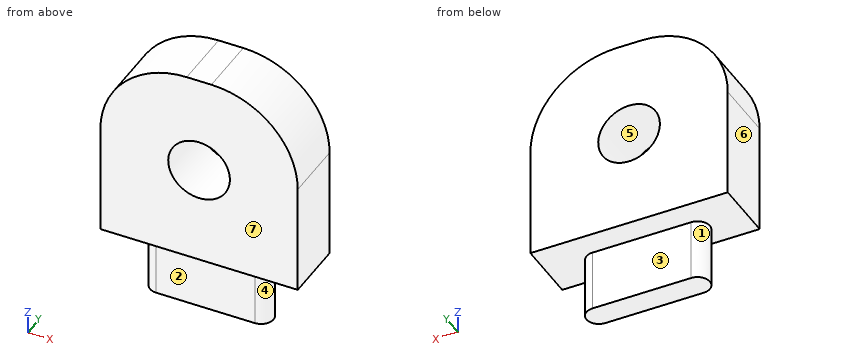
from build123d import *

# Parameters (mm, degrees)
SKETCH1_R           = 2.5
BOSS_EXTRUDE1_DEPTH = 5
BOSS_EXTRUDE2_DEPTH = 5


with BuildPart() as part:
    # Sketch1 → Boss-Extrude1 (new body)
    with BuildSketch(Plane(origin=(0, 0, 0), x_dir=(1, 0, 0), z_dir=(0, 1, 0))):
        with BuildLine():
            Line((-8, 0), (-8, -9))
            ThreePointArc((-8, -9), (-5.949747468, -13.949747468), (-1, -16))
            Line((-1, -16), (1, -16))
            ThreePointArc((1, -16), (5.949747468, -13.949747468), (8, -9))
            Line((8, -9), (8, 0))
            Line((8, 0), (-8, 0))
        make_face()
        with Locations(Location((0, -8, 0), (0, 0, 270))):
            Circle(SKETCH1_R, mode=Mode.SUBTRACT)
    extrude(amount=BOSS_EXTRUDE1_DEPTH)

    # Sketch2 → Boss-Extrude2 (add)
    with BuildSketch(Plane(origin=(0, 0, 0), x_dir=(-1, 0, 0), z_dir=(0, 0, -1))):
        with BuildLine():
            Line((-4, 3), (4, 3))
            ThreePointArc((4, 3), (5, 2), (4, 1))
            Line((4, 1), (-4, 1))
            ThreePointArc((-4, 1), (-5, 2), (-4, 3))
        make_face()
    extrude(amount=BOSS_EXTRUDE2_DEPTH)


solid = part.part
Could you check a few things on this model? Use its own coordinates, in mm. Face numbers are marked on the shaded views. A direction names the side the tool comes from. Coordinates: 2 decimals unless noted, no trailing zeros. Order: outer loops, then holes, each group sorted by start corner. A loop starts at its lowest first (then second) coordinate and runs counter-clockwise, first axis right, second up.
Q1. Suppose I cut it at C-C on x = 1.25. Please give me the cut outline in (y, z).
Q2. Which directions (+Z, -Z, +X, -X, +Y, -Y) give clear straight access to the entire face, cutting with the end or side of a thin tool? Please do the marked faces 1, 2 and 3.
Q3. Suppose I cut it at D-D on z = 5.75. Please give me the cut outline in (x, y).
Q4. Please list where these lines run through material, in increasing order: L1, parallel to X at y = 3.6, z = 8; L2, parallel to Z at x = 1.75, y = 3.15; L3, parallel to X at y = 2.35, z = 7.
Q5. Thinking about a two-plate mould opening in X: for the marked faces 4, 5, 6 and 7, which applies, released by +X, released by -X, zero draft, split by the parting line, or undercut?
Q6. Suppose I cut it at B-B on y = 2. Please give me the cut outline in (x, z).
Q7. Will these pins go through, and if not, where does the flat tip stop? pin 1 (1.5 mm diameter, centred on x = 5, y = 4.5, fed in from +Z); pin 2 (1 mm diameter, centred on x = 5.5, y = 0.5, fed in from +Z); pin 3 (1 mm diameter, centred on y = 1, z = 12, fed in from +X).
Q8. Suppose I cut it at A-A on z = 8. Please give me the cut outline in (x, y).
Answer:
1. outline: (0, 0) - (1, 0) - (1, -5) - (3, -5) - (3, 0) - (5, 0) - (5, 5.83) - (0, 5.83) - close; (0, 10.17) - (5, 10.17) - (5, 16) - (0, 16) - close
2. face 1: -Z, -X
2. face 2: -Z, +X, -X, -Y
2. face 3: -Z, +X, -X, +Y
3. outline: (-8, 0) - (-1.09, 0) - (-1.09, 5) - (-8, 5) - close; (1.09, 0) - (8, 0) - (8, 5) - (1.09, 5) - close
4. L1: x = -8 to -2.5, 2.5 to 8
4. L2: z = 0 to 6.21, 9.79 to 15.96
4. L3: x = -8 to -2.29, 2.29 to 8
5. face 4: released by +X
5. face 5: undercut
5. face 6: released by -X
5. face 7: zero draft
6. outline: (-8, 0) - (-5, 0) - (-5, -5) - (5, -5) - (5, 0) - (8, 0) - (8, 9) arc R7 ccw to (1, 16) - (-1, 16) arc R7 ccw to (-8, 9) - close; hole circle Ø5 at (0, 8)
7. pin 1: stops at z = 15.2
7. pin 2: stops at z = 14.74
7. pin 3: stops at x = 7.54
8. outline: (-8, 0) - (-2.5, 0) - (-2.5, 5) - (-8, 5) - close; (2.5, 0) - (8, 0) - (8, 5) - (2.5, 5) - close
